Source: three-view drawing plus pictorial views. Frame: mm from the lowest corner of the part. Give positions to 0.01 mm unless a question says otherwise; leave off trailing zeros. Order: outer loops, then holes, each group sorted by start corner. A loop starts at its lowest first (then second) coordinate and runs counter-clockwise, first axis right, second up. Notation, with made-up numbers: M -8.75,-16 L 5.25,-16 A6 cw 5.25,-8 Z; hole C -35.75,25.5 d4. An arc over 180 degrees is marked long. Use CSV: the item, a comma, the result in double quotes. Start each with the question number.
1. Pin query (flat end, axial travel): P1, Ø1.5, axis at y = 6.5, z = 40.5, coming from the +X side; P2, Ø2, axis at y = 2, z = 32.5, coming from the -X side; P3, Ø2.5, axis at x = 4, y = 4, coming from the +Z side. Return the tip coordinate at first contact, or that it passes through.
2. Section query C-C, the plane z = 22.5. Return the cut outline in (x, y).
3. Section query D-D, the plane x = 0.5. Return the cut outline in (y, z).
4. Line query: line 1 along Y through (x, z) = (4, 43); line 2 along Z through (x, y) = (3.5, 4.5); line 3 along Y through (x, z) = (3.5, 16). Output: solid intervals per line, ascending. Write a range as [from, to].
5. Section query A-A, the plane x = 4. Return the cut outline in (y, z), plus the area to 3 significant figures.
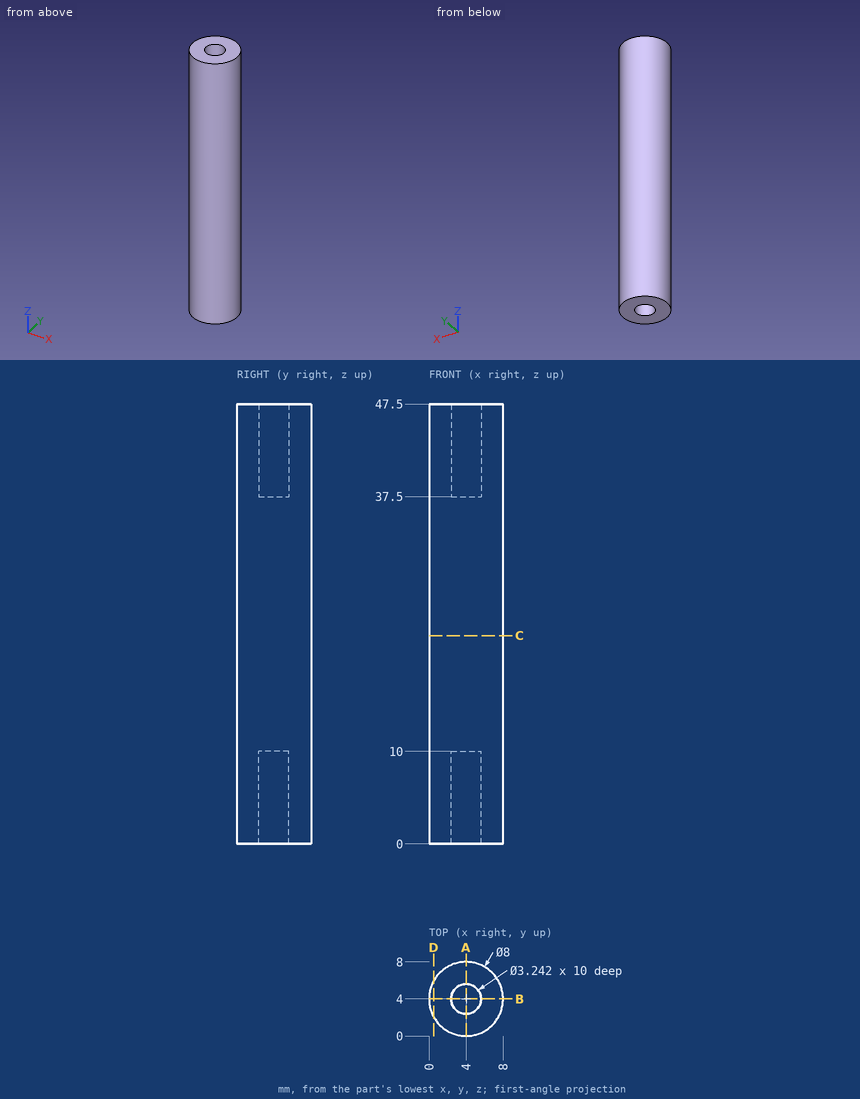
Result set:
1,P1,"x = 7.6"
1,P2,"x = 0.13"
1,P3,"z = 37.5"
2,outline,"C 4,4 d8"
3,outline,"M 2.06,0 L 5.94,0 L 5.94,47.5 L 2.06,47.5 Z"
4,line 1,"[0, 2.38], [5.62, 8]"
4,line 2,"[10, 37.5]"
4,line 3,"[0.03, 7.97]"
5,outline,"M 0,0 L 2.38,0 L 2.38,10 L 5.62,10 L 5.62,0 L 8,0 L 8,47.5 L 5.62,47.5 L 5.62,37.5 L 2.38,37.5 L 2.38,47.5 L 0,47.5 Z"
5,area,"315 mm2"
